```python
from build123d import *

# Parameters (mm, degrees)
ESBO_O1_W                = 8
ESBO_O1_H                = 9.5
RESSALTO_EXTRUS_O1_DEPTH = 18.5
ESBO_O2_R                = 0.625
ESBO_O2_R_2              = 0.25
RESSALTO_EXTRUS_O2_DEPTH = 220
CORTE_EXTRUS_O1_START    = -230
ESBO_O2_3_R              = 0.25
CORTE_EXTRUS_O1_DEPTH    = 230


with BuildPart() as part:
    # Esboço1 → Ressalto-extrusão1 (new body)
    with BuildSketch(Plane.XY):
        Rectangle(ESBO_O1_W, ESBO_O1_H)
    extrude(amount=RESSALTO_EXTRUS_O1_DEPTH)

    # Esboço2 → Ressalto-extrusão2 (add)
    with BuildSketch(Plane.XY.offset(18.5)):
        Circle(ESBO_O2_R)
        Circle(ESBO_O2_R_2, mode=Mode.SUBTRACT)
    extrude(amount=RESSALTO_EXTRUS_O2_DEPTH)

    # Esboço2<3> → Corte-extrusão1 (cut)
    with BuildSketch(Plane.XY.offset(18.5).offset(CORTE_EXTRUS_O1_START)):
        Circle(ESBO_O2_3_R)
    extrude(amount=CORTE_EXTRUS_O1_DEPTH, mode=Mode.SUBTRACT)


solid = part.part
```
The listing builds one solid part. Answer for the finished solid, in the listing's coordinates (mm). Give positions to 0.01 mm unless a question says otherwise; leave off trailing zeros. Loops run counter-clockwise (first coordinate to the right, second up) from the corner with the lowest first, then second, coordinate; pieces in that order, holes last. Notation, with made-up numbers: (33.25, 54.5) - (59.25, 54.5) arc R18 cw to (59.25, 73.5) - close; hole circle Ø3 at (63.5, 52.25). An arc over 180 degrees is marked (long way). Return JSON: item names as keys, results as strings. Group by question number.
1. Find section B-B (x = 2.5). Write down the section's boundary in (y, z).
2. Straight lines are drawn through the part: line 1 (Y direction, x = 0, z = 170.5) (3 decimals); line 2 (Z direction, x = 2.75, y = -4); line 3 (Y direction, x = -0.5, z = 158.5) (3 decimals). For each, find the intervals that lie inside material, in ascending order. Write a range as [from, to].
3. Find section A-A (y = -2.75). Write down the section's boundary in (x, z).
4. Find section C-C (z = 177). Write down the section's boundary in (x, y) (3 decimals), then the cut area to 3 significant figures.
5. Given pin 1 Ø3 at (x, y) = (-0.5, -3.5) entering from +Z; pin 2 Ø5 at (y, z) = (-1, 83.5) entering from +X (3 decimals), each flat-ended and moving along its own axis, determine where each tip first touches the part or whether it passes through.
Verdict:
{
 "1": {"outline": "(-4.75, 0) - (4.75, 0) - (4.75, 18.5) - (-4.75, 18.5) - close"},
 "2": {"line 1": "y = [-0.625, -0.25], [0.25, 0.625]", "line 2": "z = [0, 18.5]", "line 3": "y = [-0.375, 0.375]"},
 "3": {"outline": "(-4, 0) - (4, 0) - (4, 18.5) - (-4, 18.5) - close"},
 "4": {"outline": "circle Ø1.25 at (0, 0); hole circle Ø0.5 at (0, 0)", "area": "1.03 mm^2"},
 "5": {"pin 1": "stops at z = 18.5", "pin 2": "stops at x = 0.625"}
}
